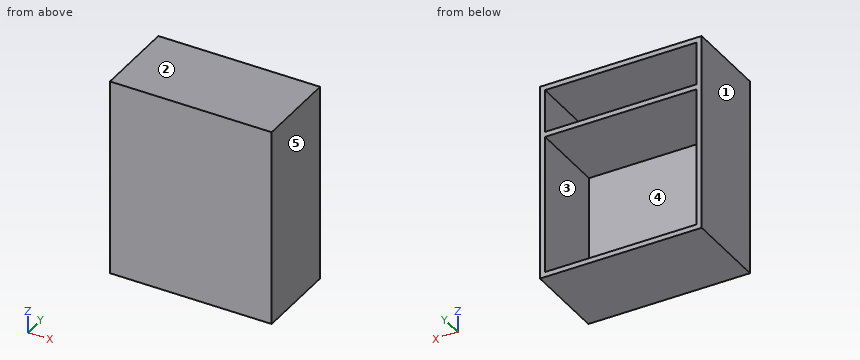
from build123d import *

# Parameters (mm, degrees)
BOSS_EXTRUDE1_DEPTH = 30
SKETCH4_W           = 63.79
SKETCH4_H           = 78
BOSS_EXTRUDE2_DEPTH = 3


with BuildPart() as part:
    # Sketch2 → Boss-Extrude1 (new body)
    with BuildSketch(Plane(origin=(0, 0, 0), x_dir=(1, 0, 0), z_dir=(0, 1, 0))):
        Polygon((-27.215737325, -52.730163819), (-29.215737325, -52.730163819), (-29.215737325, -71.730163819), (34.574262675, -71.730163819), (34.574262675, -52.730163819), (32.574262675, -52.730163819), (32.574262675, -69.730163819), (-27.215737325, -69.730163819), align=None)
        Polygon((-29.215737325, -50.730163819), (-27.215737325, -50.730163819), (-27.215737325, 4.269836181), (32.574262675, 4.269836181), (32.574262675, -50.730163819), (34.574262675, -50.730163819), (34.574262675, 6.269836181), (-29.215737325, 6.269836181), align=None)
        Polygon((32.574262675, -50.730163819), (-27.215737325, -50.730163819), (-29.215737325, -50.730163819), (-29.215737325, -52.730163819), (-27.215737325, -52.730163819), (32.574262675, -52.730163819), (34.574262675, -52.730163819), (34.574262675, -50.730163819), align=None)
    extrude(amount=BOSS_EXTRUDE1_DEPTH)

    # Sketch4 → Boss-Extrude2 (add)
    with BuildSketch(Plane.XZ):
        with Locations((2.679262675, 32.730163819)):
            Rectangle(SKETCH4_W, SKETCH4_H)
    extrude(amount=BOSS_EXTRUDE2_DEPTH)


solid = part.part
The model under review builds one solid part; all positions refer to its coordinate system, in mm. Face numbers are marked on the shaded views. A direction names the side the tool comes from. Round coordinates to 2 decimals unless told otherwise and drop trailing zeros. Write each loop counter-clockwise with the first axis right and the second up, starting at its lowest first coordinate (ties: lowest second). Pieces come first, ordered by that corner, then holes. Notation, with made-up numbers: M -10,67.5 L 28,67.5 A5 cw 28,76.5 Z; hole C 32.5,-40 d10. An arc over 180 degrees is marked long. Answer as CSV lines item,"result". Start each with the question number.
Q1. The part is to be moulded in two halves that separate along X. For the marked faces 1, 2 and 3, say which applies: +X half, -X half, draft (parallel to the pull), parting line (faces both ways), or undercut.
Q2. Tool access review of the marked faces 4 and 5: name each direction out of +Z, -Z, +X, -X, +Y, -Y from which nothing blocks a thin tool from reaching the whole face with its end or side.
Q3. Wall thickness on line 1 along Z through (x, y) = (-2, 2.5); line 2 along X through (y, z) = (8.5, 42); line 3 along Y through (x, z) = (-11, 4): over which ranges is each line inside the solid? List them lowest first.
Q4. Consider section A-A, the plane y = 24.5. Give the boundary of the cut face in (x, z), then the cut area to 3 significant figures.
Q5. Clearance check with a flat-ended pin moving along its axis: P1, Ø10, axis at x = 3.5, z = 33, coming from the +Y side. State where the tip first meets the part, or that it passes through.
Q6. Consider section C-C, the plane x = 14. Give the boundary of the cut face in (y, z).
Q7. Consider section B-B, the plane z = 46. Give the boundary of the cut face in (x, y).
Result set:
1,face 1,"-X half"
1,face 2,"draft"
1,face 3,"undercut"
2,face 4,"+Y"
2,face 5,"+Z, -Z, +X, +Y, -Y"
3,line 1,"z = -6.27 to -4.27, 50.73 to 52.73, 69.73 to 71.73"
3,line 2,"x = -29.22 to -27.22, 32.57 to 34.57"
3,line 3,"y = -3 to 0"
4,outline,"M -29.22,-6.27 L 34.57,-6.27 L 34.57,71.73 L -29.22,71.73 Z; hole M -27.22,-4.27 L 32.57,-4.27 L 32.57,50.73 L -27.22,50.73 Z; hole M -27.22,52.73 L 32.57,52.73 L 32.57,69.73 L -27.22,69.73 Z"
4,area,"671 mm²"
5,P1,"stops at y = 0"
6,outline,"M -3,-6.27 L 30,-6.27 L 30,-4.27 L 0,-4.27 L 0,50.73 L 30,50.73 L 30,52.73 L 0,52.73 L 0,69.73 L 30,69.73 L 30,71.73 L -3,71.73 Z"
7,outline,"M -29.22,-3 L 34.57,-3 L 34.57,30 L 32.57,30 L 32.57,0 L -27.22,0 L -27.22,30 L -29.22,30 Z"
